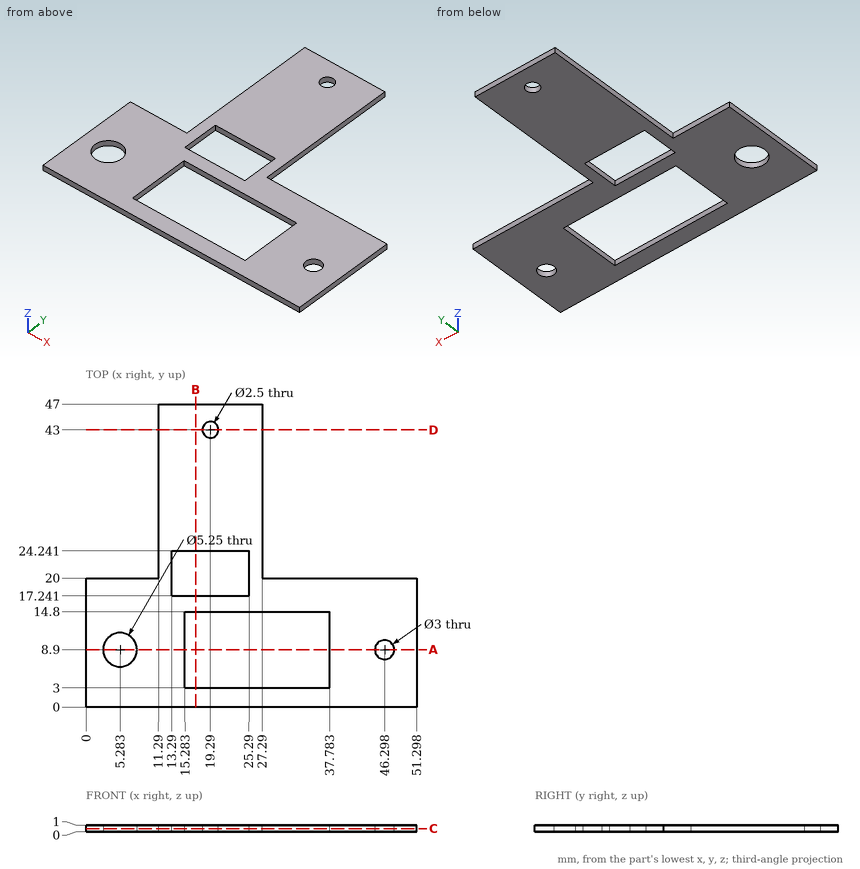
Source: three-view drawing plus pictorial views. Frame: mm from the lowest corner of the part. Round coordinates to 2 decimals unless told otherwise and drop trailing zeros. Loops run counter-clockwise (first coordinate to the right, second up) from the corner with the lowest first, then second, coordinate; pieces in that order, holes last.
Q1. Section A-A on y = 8.9. Return loops of the section in (x, z).
Q2. Section B-B on x = 17. Return loops of the section in (y, z).
Q3. Section C-C on z = 0.45. State how many separate pieces and enclosed holes the cut face has, plus the area to 4 significant figures.
Q4. Material intervals for L1, parallel to Y at x = 24.5, z = 0.35; L2, parallel to X at y = 9, z = 0.1 (1 decimal); L3, parallel to Y at x = 14, z = 0.3, sorted ascending.
Q5. Section D-D on y = 43. Return loops of the section in (x, z).
Q6. Pin query (flat end, axial travel): P1, Ø2.5, axis at x = 46.3, y = 8.9, coming from the -Z side; P2, Ø4, axis at x = 19.29, y = 43, coming from the +Z side; P3, Ø0.5, axis at y = 28.5, z = 0.5, coming from the +X side; P4, Ø0.5, axis at x = 32, z = 0.5, coming from the +Y side. Return the tip coordinate at first contact, or that it passes through.
Evaluation:
1. outline: (0, 0) - (2.66, 0) - (2.66, 1) - (0, 1) - close; (7.91, 0) - (15.28, 0) - (15.28, 1) - (7.91, 1) - close; (37.78, 0) - (44.8, 0) - (44.8, 1) - (37.78, 1) - close; (47.8, 0) - (51.3, 0) - (51.3, 1) - (47.8, 1) - close
2. outline: (0, 0) - (3, 0) - (3, 1) - (0, 1) - close; (14.8, 0) - (17.24, 0) - (17.24, 1) - (14.8, 1) - close; (24.24, 0) - (47, 0) - (47, 1) - (24.24, 1) - close
3. separate pieces: 1
3. enclosed holes: 5
3. area: 1,075 mm2
4. L1: y = 0 to 3, 14.8 to 17.24, 24.24 to 47
4. L2: x = 0 to 2.7, 7.9 to 15.3, 37.8 to 44.8, 47.8 to 51.3
4. L3: y = 0 to 17.24, 24.24 to 47
5. outline: (11.29, 0) - (18.04, 0) - (18.04, 1) - (11.29, 1) - close; (20.54, 0) - (27.29, 0) - (27.29, 1) - (20.54, 1) - close
6. P1: passes through
6. P2: stops at z = 1
6. P3: stops at x = 27.29
6. P4: stops at y = 20
